```python
from build123d import *

# Parameters (mm, degrees)
F0_R     = 28.5
F0_R_2   = 11
F1_DEPTH = 17.5
F2_R     = 10
F3_SIZE  = 5


with BuildPart() as f1:
    # F0 (on Front) → F1 (new body, symmetric)
    with BuildSketch(Plane.XZ):
        Circle(F0_R)
        Circle(F0_R_2, mode=Mode.SUBTRACT)
    extrude(amount=F1_DEPTH, both=True)

    # F2
    f2_edges = [f1.edges().sort_by_distance(p)[0] for p in [
        (-28.5, -17.5, 0),
        (-28.5, 17.5, 0),
    ]]
    fillet(f2_edges, radius=F2_R)

    # F3
    f3_edges = [f1.edges().sort_by_distance(p)[0] for p in [
        (28.5, 0, 0),
        (-28.5, 7.5, 0),
        (-28.5, -7.5, 0),
        (-11, -17.5, 0),
        (-11, 17.5, 0),
    ]]
    chamfer(f3_edges, length=F3_SIZE)


solid = f1.part
```
Can you work these out from the model? Positions are in its coordinate system, mm. Coordinates: 2 decimals unless noted, no trailing zeros. Loops run counter-clockwise (first coordinate to the right, second up) from the corner with the lowest first, then second, coordinate; pieces in that order, holes last.
Item 1: Suppose I cut it at A-A (x = 0). Please give me the cut outline in (y, z).
Answers below:
outline: (-17.5, -18.5) arc R10 ccw to (-7.5, -28.5) - (7.5, -28.5) arc R10 ccw to (17.5, -18.5) - (17.5, -16) - (12.5, -11) - (-12.5, -11) - (-17.5, -16) - close; (-17.5, 16) - (-12.5, 11) - (12.5, 11) - (17.5, 16) - (17.5, 18.5) arc R10 ccw to (7.5, 28.5) - (-7.5, 28.5) arc R10 ccw to (-17.5, 18.5) - close
Item 2: I'm going to push flat-ended pins straight in: pin 1 (5 mm diameter, centred on y = -14, z = 15, fed in from -X); pin 2 (12 mm diameter, centred on x = -14.5, y = 1, fed in from +Z); pin 3 (5 mm diameter, centred on x = -9, z = -20.5, fed in from +Y). Where does each tip first touch, or does it pass through?
Answers below:
pin 1: stops at x = -23.89
pin 2: stops at z = 27.2
pin 3: stops at y = 17.4
Item 3: Suppose I cut it at C-C (y = -6). Please give me the cut outline in (x, z), then the cut area to 3 significant figures.
Answers below:
outline: circle Ø57 at (0, 0); hole circle Ø22 at (0, 0)
area: 2,170 mm2
Item 4: Suppose I cut it at D-D (y = -11.5). Please give me the cut outline in (x, z), then the cut area to 3 significant figures.
Answers below:
outline: circle Ø55.33 at (0, 0); hole circle Ø22 at (0, 0)
area: 2,020 mm2
Item 5: Please list where these lines run through material, in increasing order: L1, parallel to Z at x = 0, y = -0.75; L2, parallel to Z at x = -1, y = -15.5; L3, parallel to X at y = 11.5, z = -2.
Answers below:
L1: z = -28.5 to -11, 11 to 28.5
L2: z = -24.48 to -13.96, 13.96 to 24.48
L3: x = -27.59 to -10.82, 10.82 to 27.59
Item 6: Suppose I cut it at B-B (z = 0). Please give me the cut outline in (x, y).
Answers below:
outline: (-28.5, -7.5) arc R10 ccw to (-18.5, -17.5) - (-16, -17.5) - (-11, -12.5) - (-11, 12.5) - (-16, 17.5) - (-18.5, 17.5) arc R10 ccw to (-28.5, 7.5) - close; (11, -12.5) - (16, -17.5) - (18.5, -17.5) arc R10 ccw to (28.5, -7.5) - (28.5, 7.5) arc R10 ccw to (18.5, 17.5) - (16, 17.5) - (11, 12.5) - close
Item 7: If we mould it in two halves opening along X, with no side actions, what happens to faces 1 (the face through (-2.437, -12.743, -10.975)), 2 (the face through (-6, -17.5, 15)), 3 (the face through (26.327, -0.105, -10.916)), 4 (the face through (-2.38, 0.18, -10.74))? For each: released by +X, released by -X, zero draft, split by the parting line, or undercut.
Answers below:
face 1: undercut
face 2: zero draft
face 3: split by the parting line
face 4: undercut
